Read the model definition and answer for the solid it produces. Units are mm, in the model's axes. A direction names the side the tool comes from. Coordinates: 2 decimals unless noted, no trailing zeros. Order: outer loops, then holes, each group sorted by start corner. A loop starts at its lowest first (then second) coordinate and runs counter-clockwise, first axis right, second up. Notation, with made-up numbers: M 79.5,-14.75 L 134.5,-14.75 A27 ccw 134.5,19.25 Z; hole C 15,45 d11. An arc over 180 degrees is marked long. Write each question's results on one line, items separated by ' | '.
Autodesk Inventor part; units mm, degrees
ref_plane "YZ Plane" through (0, 0, 0) normal (1, 0, 0) x (0, 1, 0)
ref_plane "XZ Plane" through (0, 0, 0) normal (0, 1, 0) x (-1, 0, 0)
ref_plane "XY Plane" through (0, 0, 0) normal (0, 0, 1) x (1, 0, 0)
sketch "Sketch1" plane through (0, 0, 0) normal (0, 0, 1) x (1, 0, 0)
  line L0 (-40, 7.5) -> (0, 7.5)
  line L1 (0, 7.5) -> (0, -7.5)
  line L2 (0, -7.5) -> (-40, -7.5)
  line L3 (-40, -7.5) -> (-40, 7.5)
  line L4 (-15, 52.5) -> (0, 52.5)
  line L5 (0, 52.5) -> (0, 7.5)
  line L6 (0, 7.5) -> (-15, 7.5)
  line L7 (-15, 7.5) -> (-15, 52.5)
  point P0 (0, 0)
  point P1 (-15, 7.5)
  dimension "d0" = 15
  dimension "d1" = 40
  dimension "d2" = 60
extrude "Extrusion1" add sketch "Sketch1" along normal blind 40
sketch "Sketch2" plane through (-15, 7.5, 0) normal (-1, 0, 0) x (0, 0, 1)
  line L0 (8.5, 15) -> (11.5, 15) construction
  line L1 (8.5, 12) -> (11.5, 12)
  line L2 (11.5, 18) -> (8.5, 18)
  arc A0 (8.5, 18) -> (8.5, 12) centre (8.5, 15) ccw
  arc A1 (11.5, 12) -> (11.5, 18) centre (11.5, 15) ccw
  line L3 (0, 45) -> (0, 0)
  line L4 (0, 45) -> (40, 45)
  line L5 (20, 21.547) -> (20, 15) construction
  line L6 (31.5, 15) -> (28.5, 15) construction
  line L7 (31.5, 12) -> (28.5, 12)
  line L8 (28.5, 18) -> (31.5, 18)
  arc A2 (31.5, 12) -> (31.5, 18) centre (31.5, 15) ccw
  arc A3 (28.5, 18) -> (28.5, 12) centre (28.5, 15) ccw
  point P0 (0, -7.5)
  point P1 (10, 15)
  point P2 (20, 18.2735)
  point P3 (20, 45)
  point P4 (30, 15)
  dimension "d5" = 6
  dimension "d6" = 3
  dimension "d7" = 10
  dimension "d8" = 30
extrude "Extrusion2" cut sketch "Sketch2" against normal through all
sketch "Sketch3" plane through (-40, 7.5, 0) normal (0, 1, 0) x (1, 0, 0)
  line L0 (10, -8.5) -> (10, -11.5) construction
  line L1 (7, -8.5) -> (7, -11.5)
  line L2 (13, -11.5) -> (13, -8.5)
  arc A0 (13, -8.5) -> (7, -8.5) centre (10, -8.5) ccw
  arc A1 (7, -11.5) -> (13, -11.5) centre (10, -11.5) ccw
  line L3 (25, 0) -> (0, 0)
  line L4 (0, 0) -> (0, -40)
  line L5 (15.2557, -20) -> (9.287, -20) construction
  line L6 (10, -31.5) -> (10, -28.5) construction
  line L7 (7, -31.5) -> (7, -28.5)
  line L8 (13, -28.5) -> (13, -31.5)
  arc A2 (7, -31.5) -> (13, -31.5) centre (10, -31.5) ccw
  arc A3 (13, -28.5) -> (7, -28.5) centre (10, -28.5) ccw
  point P0 (40, 0)
  point P1 (10, -10)
  point P2 (12.2713, -20)
  point P3 (0, -20)
  point P4 (10, -30)
  dimension "d11" = 3
  dimension "d12" = 6
  dimension "d13" = 10
  dimension "d14" = 10
extrude "Extrusion3" cut sketch "Sketch3" against normal through all
sketch "Sketch5" plane through (0, 0, 0) normal (0, 0, -1) x (-1, 0, 0)
  line L0 (0, -7.5) -> (15, -7.5)
  line L1 (15, -7.5) -> (15, 52.5)
  line L2 (15, 52.5) -> (0, 52.5)
  line L3 (0, 52.5) -> (0, -7.5)
  line L4 (0, -7.5) -> (0, 52.5)
  line L5 (40, -7.5) -> (0, -7.5)
  line L6 (0, 52.5) -> (15, 52.5)
  line L7 (15, 52.5) -> (15, 7.5)
  point P0 (0, 0)
  point P1 (10, 15)
extrude "Extrusion4" add sketch "Sketch5" along normal blind 30
sketch "Sketch6" plane through (0, -7.5, 40) normal (1, 0, 0) x (0, 0, -1)
  circle A0 centre (52.5, 14) radius 3
  circle A1 centre (52.5, 46) radius 3
  line L0 (70, 0) -> (0, 0)
  line L1 (70, 60) -> (70, 0)
  circle A2 centre (52.5, 30) radius 6.5
  point P0 (40, 7.5)
  dimension "d23" = 32
  dimension "d24" = 14
  dimension "d25" = 17.5
  dimension "d26" = 6
  dimension "d31" = 13
  dimension "d32" = 16
extrude "Extrusion5" cut sketch "Sketch6" against normal through all
sketch "Sketch7" plane through (0, 0, 40) normal (0, 0, 1) x (1, 0, 0)
  line L0 (0, 52.5) -> (-15, 52.5)
  line L1 (-15, 52.5) -> (-15, -7.5)
  line L2 (-15, -7.5) -> (0, -7.5)
  line L3 (0, -7.5) -> (0, 52.5)
  line L4 (0, -7.5) -> (0, 52.5)
  line L5 (0, 52.5) -> (-15, 52.5)
  line L6 (-15, 52.5) -> (-15, 7.5)
  line L7 (-40, -7.5) -> (0, -7.5)
  point P0 (0, 0)
  point P1 (-10, 15)
extrude "Extrusion6" add sketch "Sketch7" along normal blind 35
sketch "Sketch8" plane through (0, -7.5, -30) normal (1, 0, 0) x (0, 0, -1)
  circle A0 centre (-85.5, 30) radius 6
  circle A1 centre (-85.5, 17) radius 3
  circle A2 centre (-85.5, 43) radius 3
  line L0 (-105, 60) -> (0, 60)
  line L1 (-105, 0) -> (-105, 60)
  point P0 (-30, 7.5)
  dimension "d33" = 12
  dimension "d34" = 6
  dimension "d35" = 17
  dimension "d36" = 19.5
  dimension "d37" = 26
  dimension "d38" = 13
extrude "Extrusion7" cut sketch "Sketch8" against normal through all
chamfer "Chamfer2" distance 5 angle 45 3 edges at (-15, 0, 40) (-15, 7.5, 20) (-15, 0, 0)
fillet "Fillet2" radius 5 4 edges at (-7.5, 52.5, 75) (-7.5, -7.5, 75) (-7.5, 52.5, -30) (-7.5, -7.5, -30)
equation "\"d32\" = 0.5 * d23"
equation "\"d38\" = 0.5 * d37"
properties part number "0008-10-033" material "ABS Plastic"
(1) The part is cut by section B-B, the plane x = -9. Count the separate pieces of the cut face and the enclosed holes in it, then the cut area to 3 significant figures.
Conclusion:
separate pieces: 1 | enclosed holes: 8 | area: 5,830 mm²
(2) The mould has two halves that part along Z. Classify faces 1 (the flat face through (-30, 0, 40)), 2 (the flat face through (-7, 23, -30)), 3 (the cylindrical face through (-7.395, 22.764, 61.494)), 4 (the flat face through (-16, -7.5, 22)): pulls with the +Z half, pulls with the -Z half, needs draft (parallel to the pull), parting line crosses it, or undercut.
Conclusion:
face 1: pulls with the +Z half | face 2: pulls with the -Z half | face 3: undercut | face 4: needs draft
(3) Given pin 1 (8 mm diameter, centred on x = -32.5, z = 23.5, fed in from +Y); pin 2 (1 mm diameter, centred on y = 18.5, z = 60.5, fed in from -X); pin 3 (12 mm diameter, centred on x = -33.5, y = 1, fed in from -Z), each flat-ended and moving along its own axis, determine where each tip first touches the part or whether it passes through.
Conclusion:
pin 1: y = 7.5 | pin 2: x = -15 | pin 3: z = 0
(4) The part is cut by section C-C, the plane x = -30. Write down the section's boundary in (y, z), then the cut area to 3 significant figures.
Conclusion:
outline: M -7.5,0 L 7.5,0 L 7.5,5.5 L -7.5,5.5 Z; M -7.5,14.5 L 7.5,14.5 L 7.5,25.5 L -7.5,25.5 Z; M -7.5,34.5 L 7.5,34.5 L 7.5,40 L -7.5,40 Z | area: 330 mm²
(5) Straight lines are drawn through the part: line 1 (Y direction, x = -5, z = 55.5); line 2 (Z direction, x = -11, y = 38); line 3 (X direction, y = 19, z = 38.5). For each, find the intervals that lie inside material, in ascending order.
Conclusion:
line 1: -7.5 to 6.5, 12.5 to 16.5, 28.5 to 32.5, 38.5 to 52.5 | line 2: -30 to -15.46, -9.54 to 53.84, 57.16 to 75 | line 3: -15 to 0
(6) The part is cut by section A-A, the plane y = 22.5. Write down the section's boundary in (x, z), then the cut area to 3 significant figures.
Conclusion:
outline: M -15,-30 L 0,-30 L 0,-19 L -15,-19 Z; M -15,-6 L 0,-6 L 0,5.5 L -15,5.5 Z; M -15,14.5 L 0,14.5 L 0,25.5 L -15,25.5 Z; M -15,34.5 L 0,34.5 L 0,49.5 L -15,49.5 Z; M -15,61.5 L 0,61.5 L 0,75 L -15,75 Z | area: 930 mm²
(7) For faces 5 (the flat face through (-30, 7.5, 20)), 6 (the cylindrical face through (-7.6, 51, 73.57)), 7 (the flat face through (-8, 19.5, 10)), 8 (the flat face through (-33, 0, 10)), 9 (the flat face through (-7, 52.5, 22)), determine the directions among +Z, -Z, +X, -X, +Y, -Y from which every point of the face is accessible in a straight line to the end or side of a thin tool.
Conclusion:
face 5: +Z, -Z, -X, +Y | face 6: +Z, +X, -X, +Y | face 7: +X, -X | face 8: +Y, -Y | face 9: +Z, -Z, +X, -X, +Y
(8) The part is cut by section D-D, the plane y = 34. Write down the section's boundary in (x, z).
Conclusion:
outline: M -15,-30 L 0,-30 L 0,52.9 L -15,52.9 Z; M -15,58.1 L 0,58.1 L 0,75 L -15,75 Z
